Verification items for the finished model (mm, model axes). A direction names the side the tool comes from. Round coordinates to 2 decimals unless told otherwise and drop trailing zeros. Order: outer loops, then holes, each group sorted by start corner. A loop starts at its lowest first (then second) coordinate and runs counter-clockwise, first axis right, second up. Notation, with made-up numbers: (-0.5, 67) -> (57.5, 67) arc R11 cw to (57.5, 81) -> close; hole circle Ø7 at (61, 62). An arc over 180 degrees is marked (long way). Put each result on its own line as item: value.
from build123d import *

# Parameters (mm, degrees)
SKETCH1_W                      = 240.6
SKETCH1_H                      = 180.2
BOSS_EXTRUDE1_DEPTH            = 8
SKETCH2_W                      = 160.6
SKETCH2_H                      = 100.2
CUT_EXTRUDE1_DEPTH             = 200.503872501
CUT_EXTRUDE2_DEPTH             = 7
CUT_EXTRUDE3_DEPTH             = 7
CUT_EXTRUDE4_DEPTH             = 7
CUT_EXTRUDE5_DEPTH             = 7
F_6_5_6_5_DIAMETER_HOLE1_D     = 6.5
F_6_5_6_5_DIAMETER_HOLE1_DEPTH = 8
SKETCH9_R                      = 9.267416037
SKETCH9_R_2                    = 9.269178346
SKETCH9_R_3                    = 9.266671768
CUT_EXTRUDE7_DEPTH             = 4
BOSS_EXTRUDE2_DEPTH            = 10
BOSS_EXTRUDE3_DEPTH            = 10
BOSS_EXTRUDE4_DEPTH            = 10
BOSS_EXTRUDE5_DEPTH            = 10
SKETCH18_W                     = 10
SKETCH18_H                     = 10.641777725
SKETCH18_R                     = 1.5
BOSS_EXTRUDE6_DEPTH            = 3


with BuildPart() as part:
    # Sketch1 → Boss-Extrude1 (new body)
    with BuildSketch(Plane(origin=(0, 0, 0), x_dir=(-1, 0, 0), z_dir=(0, 0, -1))):
        with Locations((-50.702318109, 12.34999924)):
            Rectangle(SKETCH1_W, SKETCH1_H)
    extrude(amount=-BOSS_EXTRUDE1_DEPTH)

    # Sketch2 → Cut-Extrude1 (cut, through all)
    with BuildSketch(Plane.XY.offset(8)):
        with Locations((50.702318109, 12.34999924)):
            Rectangle(SKETCH2_W, SKETCH2_H)
    extrude(amount=-CUT_EXTRUDE1_DEPTH, mode=Mode.SUBTRACT)

    # Sketch3 → Cut-Extrude2 (cut)
    with BuildSketch(Plane(origin=(0, 0, 0), x_dir=(-1, 0, 0), z_dir=(0, 0, -1))):
        Polygon((-117.686768689, -48.483328992), (-127.060792146, -58.198146757), (-117.921667286, -67.016672528), (-108.547643828, -57.301854763), align=None)
    extrude(amount=-CUT_EXTRUDE2_DEPTH, mode=Mode.SUBTRACT)

    # Sketch4 → Cut-Extrude3 (cut)
    with BuildSketch(Plane(origin=(0, 0, 0), x_dir=(-1, 0, 0), z_dir=(0, 0, -1))):
        Polygon((6.939207854, -58.198146757), (16.078332714, -67.016672528), (25.452356172, -57.301854763), (16.313231311, -48.483328992), align=None)
    extrude(amount=-CUT_EXTRUDE3_DEPTH, mode=Mode.SUBTRACT)

    # Sketch5 → Cut-Extrude4 (cut)
    with BuildSketch(Plane(origin=(0, 0, 0), x_dir=(-1, 0, 0), z_dir=(0, 0, -1))):
        Polygon((-37.727458813, -58.198146757), (-28.588333952, -67.016672528), (-19.214310494, -57.301854763), (-28.353435355, -48.483328992), align=None)
    extrude(amount=-CUT_EXTRUDE4_DEPTH, mode=Mode.SUBTRACT)

    # Sketch6 → Cut-Extrude5 (cut)
    with BuildSketch(Plane(origin=(0, 0, 0), x_dir=(-1, 0, 0), z_dir=(0, 0, -1))):
        Polygon((-82.39412548, -58.198146757), (-73.255000619, -67.016672528), (-63.880977161, -57.301854763), (-73.020102022, -48.483328992), align=None)
    extrude(amount=-CUT_EXTRUDE5_DEPTH, mode=Mode.SUBTRACT)

    # Ø6.5 (6.5) Diameter Hole1
    with Locations(Plane.XY.offset(8)):
        with Locations((117.804217987, -57.75000076), (-16.097681891, -57.75000076), (28.568984776, -57.75000076), (73.235651442, -57.75000076)):
            Hole(F_6_5_6_5_DIAMETER_HOLE1_D / 2, depth=F_6_5_6_5_DIAMETER_HOLE1_DEPTH)

    # Sketch9 → Cut-Extrude7 (cut)
    with BuildSketch(Plane(origin=(0, 0, 0), x_dir=(-1, 0, 0), z_dir=(0, 0, -1))):
        with Locations((-117.804217987, -57.75000076)):
            Circle(SKETCH9_R)
        with Locations((-73.235651442, -57.75000076)):
            Circle(SKETCH9_R_2)
        with Locations((-28.568984776, -57.75000076)):
            Circle(SKETCH9_R_2)
        with Locations((16.097681891, -57.75000076)):
            Circle(SKETCH9_R_3)
    extrude(amount=-CUT_EXTRUDE7_DEPTH, mode=Mode.SUBTRACT)

    # Sketch12 → Boss-Extrude2 (add)
    with BuildSketch(Plane(origin=(171.002318109, 0, 0), x_dir=(0, 0, -1), z_dir=(1, 0, 0))):
        Polygon((0, -77.75000076), (15, -77.75000076), (22.478199259, -57.203817156), (0, -57.203817156), align=None)
    extrude(amount=-BOSS_EXTRUDE2_DEPTH)

    # Sketch14 → Boss-Extrude3 (add)
    with BuildSketch(Plane.ZY.offset(69.597681891)):
        Polygon((-22.478199259, -57.203817156), (-15, -77.75000076), (0, -77.75000076), (0, -57.203817156), align=None)
    extrude(amount=-BOSS_EXTRUDE3_DEPTH)

    # Sketch15 → Boss-Extrude4 (add)
    with BuildSketch(Plane.ZY.offset(69.597681891)):
        Polygon((0, 102.44999924), (-80.587436215, 102.44999924), (-76.947733872, 92.44999924), (0, 92.44999924), align=None)
    extrude(amount=-BOSS_EXTRUDE4_DEPTH)

    # Sketch16 → Boss-Extrude5 (add)
    with BuildSketch(Plane(origin=(171.002318109, 0, 0), x_dir=(0, 0, -1), z_dir=(1, 0, 0))):
        Polygon((0, 102.44999924), (80.587436215, 102.44999924), (76.947733872, 92.44999924), (0, 92.44999924), align=None)
    extrude(amount=-BOSS_EXTRUDE5_DEPTH)

    # Sketch18 → Boss-Extrude6 (add, along a direction that is not the sketch's normal)
    # profile 1 of 2: a face of its own
    with BuildSketch(Plane(origin=(0, -13.915929435, -38.233701894), x_dir=(-1, 0, 0), z_dir=(0, -0.3420201433256657, -0.9396926207859096))):
        with Locations((54.597681891, 118.513145908)):
            Rectangle(SKETCH18_W, SKETCH18_H)
        with Locations((54.597681891, 118.513145907)):
            Circle(SKETCH18_R, mode=Mode.SUBTRACT)
    # profile 2 of 2: a face of its own
    with BuildSketch(Plane(origin=(0, -13.915929435, -38.233701894), x_dir=(-1, 0, 0), z_dir=(0, -0.3420201433256657, -0.9396926207859096))):
        with Locations((-156.002318109, 118.513145908)):
            Rectangle(SKETCH18_W, SKETCH18_H)
        with Locations((-156.002318109, 118.513145907)):
            Circle(SKETCH18_R, mode=Mode.SUBTRACT)
    extrude(amount=-BOSS_EXTRUDE6_DEPTH, dir=(0, 0, -1))


solid = part.part
Item 1: Section check A-A on y = -6.5. Record the boundary of the cut face in (x, z), then the cut area to 3 significant figures.
Check sheet entries:
outline: (-69.6, 0) -> (-29.6, 0) -> (-29.6, 8) -> (-69.6, 8) -> close; (131, 0) -> (171, 0) -> (171, 8) -> (131, 8) -> close
area: 640 mm^2
Item 2: Gauge pin test, flat ends, axial feed: pin 1 Ø7.5 at (x, y) = (117.8, -57.75) entering from +Z; pin 2 Ø3 at (x, y) = (-21, -62.5) entering from -Z; pin 3 Ø20.5 at (x, y) = (118, -57.5) entering from -Z; pin 4 Ø5.5 at (x, y) = (76, -57) entering from -Z. Record the tip position at first contact, or that the pin passes through.
Check sheet entries:
pin 1: stops at z = 8
pin 2: stops at z = 4
pin 3: stops at z = 0
pin 4: stops at z = 7
Item 3: Section check B-B on x = 92.5. Record the boundary of the cut face in (y, z).
Check sheet entries:
outline: (-77.75, 0) -> (-37.75, 0) -> (-37.75, 8) -> (-77.75, 8) -> close; (62.45, 0) -> (102.45, 0) -> (102.45, 8) -> (62.45, 8) -> close
Item 4: Section check C-C on z = -10.5. Record the boundary of the cut face in (x, y).
Check sheet entries:
outline: (-69.6, -77.75) -> (-59.6, -77.75) -> (-59.6, -57.2) -> (-69.6, -57.2) -> close; (-69.6, 92.45) -> (-59.6, 92.45) -> (-59.6, 102.45) -> (-69.6, 102.45) -> close; (161, -77.75) -> (171, -77.75) -> (171, -57.2) -> (161, -57.2) -> close; (161, 92.45) -> (171, 92.45) -> (171, 102.45) -> (161, 102.45) -> close
Item 5: Material ranges on L1, parallel to X at y = -57.75, z = 2.2; L2, parallel to X at y = -57.75, z = 7.6; L3, parallel to Z at x = 144.5, y = -8, recorded low to high. Write a range as [from, to].
Check sheet entries:
L1: x = [-69.6, -25.36], [-6.83, 19.3], [37.84, 63.97], [82.5, 108.54], [127.07, 171]
L2: x = [-69.6, -19.35], [-12.85, 25.32], [31.82, 69.99], [76.49, 114.55], [121.05, 171]
L3: z = [0, 8]
Item 6: Tool access check on faces 4 (the flat face through (157.183, 98.631, -76.197)), 5 (the flat face through (166, -57.204, -11)), 6 (the cylindrical face through (70.136, -56.774, 7.493)), 7 (the flat face through (23.97, -62.23, 5.01)). Record the directions out of +Z, -Z, +X, -X, +Y, -Y that give a thin tool (end or side, any length) a straight path to the whole face; none if there is none.
Check sheet entries:
face 4: +Y
face 5: -Z, +X, -X
face 6: +Z, -Z
face 7: -Z
Item 7: Section check D-D on y = -42.5. Record the boundary of the cut face in (x, z), then the cut area to 3 significant figures.
Check sheet entries:
outline: (-69.6, 0) -> (171, 0) -> (171, 8) -> (-69.6, 8) -> close
area: 1,920 mm^2
Item 8: Release check for a two-part mould opening along Y. For faces 1 (the flat face through (-53.417, 98.631, -76.197)), 2 (the flat face through (68.39, -52.95, 5.01)), 3 (the flat face through (166.072, -67.621, -18.687)) record: +Y half, -Y half, draft (parallel to the pull), parting line (faces both ways), or undercut.
Check sheet entries:
face 1: +Y half
face 2: undercut
face 3: -Y half
